Verification items for the finished model (mm, model axes). Face numbers are marked on the shaded views. A direction names the side the tool comes from. Coordinates: 2 decimals unless noted, no trailing zeros. Write each loop counter-clockwise with the first axis right and the second up, starting at its lowest first coordinate (ties: lowest second). Pieces come first, ordered by that corner, then holes. Notation, with made-up numbers: (78.5, 71) -> (82.5, 71) arc R12 ccw to (82.5, 89) -> close; hole circle Ø9 at (-25.75, 55.5). An arc over 180 degrees is marked (long way). Use CSV: the item, a comma, the result in double quotes.
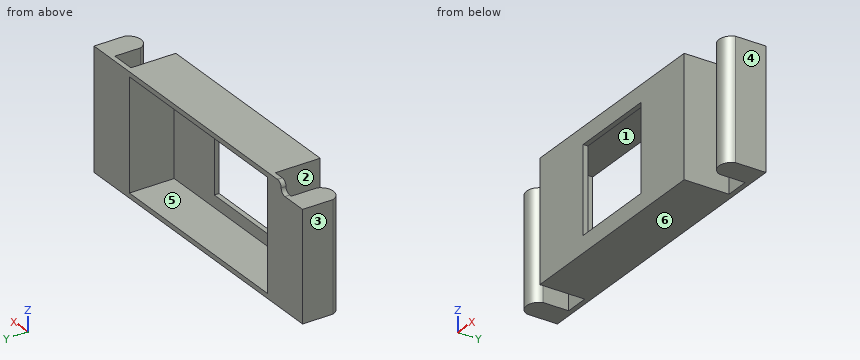
```python
from build123d import *

# Parameters (mm, degrees)
F0_W      = 60
F0_H      = 60
F0_R      = 22.4096796893
F1_DEPTH  = 3
F2_W      = 60
F2_H      = 60
F2_W_2    = 54
F2_H_2    = 54
F3_DEPTH  = 15
F4_W      = 135
F4_H      = 75
F4_W_2    = 54
F4_H_2    = 54
F5_DEPTH  = 3
F6_W      = 135
F6_H      = 75
F6_W_2    = 129
F6_H_2    = 69
F7_DEPTH  = 25
F8_W      = 195
F8_H      = 75
F8_W_2    = 129
F8_H_2    = 69
F9_DEPTH  = 3
F10_W     = 15
F10_H     = 68
F11_DEPTH = 25
F12_W     = 15
F12_H     = 75
F13_DEPTH = 25
F15_DEPTH = 200
F17_DEPTH = 25
F18_R     = 3.49999
F21_DEPTH = 60
F24_W     = 60
F24_H     = 60
F25_DEPTH = 18


# Not quite as in the source:
# - a fillet or chamfer is up to 0.001 mm smaller than in the source, because OpenCascade refuses the exact size


with BuildPart() as f1:
    # F0 (on Front) → F1 (new body)
    with BuildSketch(Plane.XZ):
        Rectangle(F0_W, F0_H)
        Circle(F0_R, mode=Mode.SUBTRACT)
    extrude(amount=F1_DEPTH)

    # F2 (on face) → F3 (join)
    with BuildSketch(Plane(origin=(0, 0, 0), x_dir=(-1, 0, 0), z_dir=(0, 1, 0))):
        Rectangle(F2_W, F2_H)
        Rectangle(F2_W_2, F2_H_2, mode=Mode.SUBTRACT)
    extrude(amount=F3_DEPTH)

    # F4 (on face) → F5 (join)
    with BuildSketch(Plane(origin=(0, 15, 0), x_dir=(-1, 0, 0), z_dir=(0, 1, 0))):
        Rectangle(F4_W, F4_H)
        Rectangle(F4_W_2, F4_H_2, mode=Mode.SUBTRACT)
    extrude(amount=F5_DEPTH)

    # F6 (on face) → F7 (join)
    with BuildSketch(Plane(origin=(0, 18, 0), x_dir=(-1, 0, 0), z_dir=(0, 1, 0))):
        Rectangle(F6_W, F6_H)
        Rectangle(F6_W_2, F6_H_2, mode=Mode.SUBTRACT)
    extrude(amount=F7_DEPTH)

    # F8 (on face) → F9 (join)
    with BuildSketch(Plane(origin=(0, 43, 0), x_dir=(-1, 0, 0), z_dir=(0, 1, 0))):
        Rectangle(F8_W, F8_H)
        Rectangle(F8_W_2, F8_H_2, mode=Mode.SUBTRACT)
    extrude(amount=F9_DEPTH)

    # F10 (on face) → F11 (join)
    with BuildSketch(Plane.XZ.offset(-43)):
        with Locations((-90, -3.5)):
            Rectangle(F10_W, F10_H)
    extrude(amount=F11_DEPTH)

    # F12 (on face) → F13 (join)
    with BuildSketch(Plane.XZ.offset(-43)):
        with Locations((90, 0)):
            Rectangle(F12_W, F12_H)
    extrude(amount=F13_DEPTH)

    # F14 (on face) → F15 (cut)
    with BuildSketch(Plane.XY.offset(37.5)):
        with BuildLine():
            ThreePointArc((-82.5, 27), (-90, 21.7838821814), (-97.5, 27))
            Line((-97.5, 27), (-97.5, 18))
            Line((-97.5, 18), (-82.5, 18))
            Line((-82.5, 18), (-82.5, 27))
        make_face()
        with BuildLine():
            ThreePointArc((97.5, 27), (90, 21.7838821814), (82.5, 27))
            Line((82.5, 27), (82.5, 18))
            Line((82.5, 18), (97.5, 18))
            Line((97.5, 18), (97.5, 27))
        make_face()
    extrude(amount=-F15_DEPTH, mode=Mode.SUBTRACT)

    # F16 (on face) → F17 (cut)
    with BuildSketch(Plane.XZ.offset(-43)):
        Polygon((-77.5, 37.5), (-82.5, 37.5), (-97.5, 37.5), (-97.5, 30.5), (-82.5, 30.5), (-77.5, 30.5), align=None)
    extrude(amount=-F17_DEPTH, mode=Mode.SUBTRACT)

    # F18 (radius 3.5 in the source; OpenCascade refuses exactly that, so slightly less here)
    f18_edges = [f1.edges().sort_by_distance(p)[0] for p in [
        (-77.5, 44.5, 30.5),
        (-77.5, 44.5, 37.5),
    ]]
    fillet(f18_edges, radius=F18_R)

    # F20 (on face) → F21 (cut)
    with BuildSketch(Plane.XY.offset(30)):
        Polygon((-30, -3), (-50, 15), (-50, -3), align=None)
    extrude(amount=-F21_DEPTH, mode=Mode.SUBTRACT)

    # F24 (on face) → F25 (cut)
    with BuildSketch(Plane.XZ.offset(3)):
        Rectangle(F24_W, F24_H)
    extrude(amount=-F25_DEPTH, mode=Mode.SUBTRACT)


solid = f1.part
```
1) Mould release check, pull along X, two halves, no side actions. Record for the marked faces 4, 5 and 6: released by +X, released by -X, zero draft, split by the parting line, or undercut.
Return value:
face 4,"released by +X"
face 5,"undercut"
face 6,"zero draft"
2) Scan lines: L1, parallel to X at y = 36, z = 11; L2, parallel to Z at x = 47, y = 21; L3, parallel to X at y = 20, z = -10.5. Record each from-to range of solid material in increasing order.
Return value:
L1,"-97.5 to -82.5, -67.5 to -64.5, 64.5 to 67.5, 82.5 to 97.5"
L2,"-37.5 to -34.5, 34.5 to 37.5"
L3,"-67.5 to -64.5, 64.5 to 67.5"
3) Cross-section at B-B (z = 10.5). Record the boundary of the cut face in (x, y).
Return value:
outline,"(-97.5, 27) arc R8 ccw to (-82.5, 27) -> (-82.5, 43) -> (-67.5, 43) -> (-67.5, 15) -> (-27, 15) -> (-27, 18) -> (-64.5, 18) -> (-64.5, 46) -> (-97.5, 46) -> close; (27, 15) -> (67.5, 15) -> (67.5, 43) -> (82.5, 43) -> (82.5, 27) arc R8 ccw to (97.5, 27) -> (97.5, 46) -> (64.5, 46) -> (64.5, 18) -> (27, 18) -> close"
4) Set-up check for the marked faces 1, 2 and 3: record each of +Z, -Z, +X, -X, +Y, -Y from which the full face is reachable in a straight line by a thin tool's end or side.
Return value:
face 1,"+Y"
face 2,"+Z, -Z, -Y"
face 3,"+Z, -Z, -X, +Y, -Y"
5) Cross-section at A-A (y = 40). Record the boundary of the cut face in (x, z), plus the area to 3 significant figures.
Return value:
outline,"(-97.5, -37.5) -> (-82.5, -37.5) -> (-82.5, 30.5) -> (-97.5, 30.5) -> close; (-67.5, -37.5) -> (67.5, -37.5) -> (67.5, 37.5) -> (-67.5, 37.5) -> close; (82.5, -37.5) -> (97.5, -37.5) -> (97.5, 37.5) -> (82.5, 37.5) -> close; hole (-64.5, -34.5) -> (64.5, -34.5) -> (64.5, 34.5) -> (-64.5, 34.5) -> close"
area,"3,370 mm2"
6) Cross-section at C-C (x = 62). Record the boundary of the cut face in (y, z), plus the area to 3 significant figures.
Return value:
outline,"(15, -37.5) -> (46, -37.5) -> (46, -34.5) -> (18, -34.5) -> (18, 34.5) -> (46, 34.5) -> (46, 37.5) -> (15, 37.5) -> close"
area,"393 mm2"
7) Gauge pin test, flat ends, axial feed: pin 1 (3.5 mm diameter, centred on y = 17, z = 4.5, fed in from +X); pin 2 (5 mm diameter, centred on x = -87.5, y = 30.5, fed in from +Z); pin 3 (1.5 mm diameter, centred on y = 16.5, z = -6, fed in from -X). Record the tip position at first contact, or that the pin passes through.
Return value:
pin 1,"x = 67.5"
pin 2,"z = 30.5"
pin 3,"x = -67.5"
8) Cross-section at D-D (y = 25). Record the boundary of the cut face in (x, z), plus the area to 3 significant figures.
Return value:
outline,"(-96.41, -37.5) -> (-83.59, -37.5) -> (-83.59, 30.5) -> (-96.41, 30.5) -> close; (-67.5, -37.5) -> (67.5, -37.5) -> (67.5, 37.5) -> (-67.5, 37.5) -> close; (83.59, -37.5) -> (96.41, -37.5) -> (96.41, 37.5) -> (83.59, 37.5) -> close; hole (-64.5, -34.5) -> (64.5, -34.5) -> (64.5, 34.5) -> (-64.5, 34.5) -> close"
area,"3,060 mm2"
